The listing builds one solid part. Answer for the finished solid, in the listing's coordinates (mm). A direction names the side the tool comes from. Round coordinates to 2 decimals unless told otherwise and drop trailing zeros. Write each loop counter-clockwise with the first axis right and the second up, starting at its lowest first coordinate (ties: lowest second). Pieces come first, ordered by that corner, then holes.
(1) The mould has two halves that part along X. Classify faces 4 (the face through (1.3, -2, 6)), 5 (the face through (1.69, 2.64, 5.24)), 6 (the face through (-0.278, 2.117, 4.768)): +X half, -X half, draft (parallel to the pull), parting line (faces both ways), or undercut.
(2) Each of these flat-tipped pins is pushed along its axis until it touches: pin 1 Ø10 at (x, y) = (-1, 0.5) entering from -Z; pin 2 Ø1 at (x, y) = (10.5, 10.5) entering from -Z; pin 3 Ø3 at (y, z) = (-9, 2.5) entering from -X; pin 4 Ø2 at (x, z) = (-8.5, 3.5) entering from -Y. Where does it stop, or does it pass through?
(3) For faces 1 (the face through (2, -2, 3)), 2 (the face through (4, 0, 4)), 3 (the face through (8, -10, 0)), determine the directions among +Z, -Z, +X, -X, +Y, -Y from which every point of the face is accessible in a straight line to the end or side of a thin tool.
(4) A cutting plane is placed at C-C, the plane z = 4.9. Give the vertices of the cut face in (x, y) (3 decimals), and give its area (3 significant figures).
(5) A cutting plane is placed at A-A, the plane y = 0. Give the vertices of the cut face in (x, z) (3 decimals).
(6) Find the intervals of material crossed by probe 1 along Y at (x, z) = (0, 5.5) (3 decimals); probe 2 along Z at (x, y) = (7, 7); probe 3 along Y at (x, z) = (0, 4.3) (3 decimals), in increasing order.
(7) A cutting plane is placed at D-D, the plane z = 1.95. Give the vertices of the cut face in (x, y), and give its area (3 significant figures).
from build123d import *

# Parameters (mm, degrees)
SKETCH1_R                      = 13.6
DRIVE_SHAFT_PLATE_SHAPE_DEPTH  = 4
PLATE_MAIN_FILLET_R            = 3.8
SKETCH2_R                      = 3.135
PLATE_BOSS_DEPTH               = 2
PLATE_SHELL_T                  = -1
DRIVE_PLATE_HOLE_REACH         = 22.147
SKETCH3_R                      = 2.135
DRIVE_PLATE_SECONDARY_FILLET_R = 0.5


with BuildPart() as part:
    # Sketch1 → drive shaft plate shape (new body)
    with BuildSketch(Plane.XY):
        Circle(SKETCH1_R)
    extrude(amount=DRIVE_SHAFT_PLATE_SHAPE_DEPTH)

    # plate main fillet
    plate_main_fillet_edges = [part.edges().sort_by_distance(p)[0] for p in [
        (-13.6, 0, 4),
    ]]
    fillet(plate_main_fillet_edges, radius=PLATE_MAIN_FILLET_R)

    # Sketch2 → plate boss (add)
    with BuildSketch(Plane.XY.offset(4)):
        Circle(SKETCH2_R)
    extrude(amount=PLATE_BOSS_DEPTH)

    # plate shell
    plate_shell_openings = [part.faces().sort_by_distance(p)[0] for p in [
        (0, 0, 0),
    ]]
    offset(amount=PLATE_SHELL_T, openings=plate_shell_openings, kind=Kind.INTERSECTION)

    # Sketch3 → drive plate hole (cut, up to next)
    with BuildSketch(Plane.XY.offset(6), mode=Mode.PRIVATE) as drive_plate_hole_sk1:
        Circle(SKETCH3_R)
    drive_plate_hole_tool1 = extrude(drive_plate_hole_sk1.sketch, amount=-DRIVE_PLATE_HOLE_REACH, mode=Mode.PRIVATE) & part.part
    add(drive_plate_hole_tool1.solids().sort_by_distance((0, 0, 6))[0], mode=Mode.SUBTRACT)

    # drive plate secondary fillet
    drive_plate_secondary_fillet_edges = [part.edges().sort_by_distance(p)[0] for p in [
        (-2.135, 0, 3),
        (-3.135, 0, 4),
    ]]
    fillet(drive_plate_secondary_fillet_edges, radius=DRIVE_PLATE_SECONDARY_FILLET_R)


solid = part.part
Solutions:
1. face 4: draft
1. face 5: parting line
1. face 6: undercut
2. pin 1: stops at z = 3
2. pin 2: passes through
2. pin 3: stops at x = -10.81
2. pin 4: stops at y = -9.9
3. face 1: -Z
3. face 2: +Z
3. face 3: -Z, +X, -X, +Y, -Y
4. outline: circle Ø6.27 at (0, 0); hole circle Ø4.27 at (0, 0)
4. area: 16.6 mm2
5. outline: (-13.6, 0) - (-12.6, 0) - (-12.6, 0.2) arc R2.8 cw to (-9.8, 3) - (-2.635, 3) arc R0.5 ccw to (-2.135, 3.5) - (-2.135, 6) - (-3.135, 6) - (-3.135, 4.5) arc R0.5 cw to (-3.635, 4) - (-9.8, 4) arc R3.8 ccw to (-13.6, 0.2) - close; (2.135, 3.5) arc R0.5 ccw to (2.635, 3) - (9.8, 3) arc R2.8 cw to (12.6, 0.2) - (12.6, 0) - (13.6, 0) - (13.6, 0.2) arc R3.8 ccw to (9.8, 4) - (3.635, 4) arc R0.5 cw to (3.135, 4.5) - (3.135, 6) - (2.135, 6) - close
6. probe 1: y = -3.135 to -2.135, 2.135 to 3.135
6. probe 2: z = 3 to 4
6. probe 3: y = -3.177 to -2.135, 2.135 to 3.177
7. outline: circle Ø26.35 at (0, 0); hole circle Ø23.97 at (0, 0)
7. area: 93.8 mm2
